For this review, take the finished solid that the model builds, in its own axes (mm). A direction names the side the tool comes from. Coordinates: 2 decimals unless noted, no trailing zeros. Loops run counter-clockwise (first coordinate to the right, second up) from the corner with the lowest first, then second, coordinate; pieces in that order, holes last. Notation, with made-up numbers: (89.5, 70) - (125.5, 70) arc R17 cw to (125.5, 74) - close; hole circle Ø7 at (77.5, -6.75). An arc over 180 degrees is marked (long way). Answer as a JSON object with one key per item and string values. Group by question number.
Item 1: We need section A-A (z = -15). Give the boundary of the cut face in (x, y), then the cut area to 3 significant figures.
Item 2: We need section B-B (y = -7.75). Give the boundary of the cut face in (x, z), then the cut area to 3 significant figures.
Item 3: We need section C-C (z = -23). Give the boundary of the cut face in (x, y), then the cut area to 3 significant figures.
Item 4: Clearance check with a flat-ended pin moving along its axis: pin 1 (5 mm diameter, centred on x = 4, y = 3, fed in from -Z). State where the tip first meets the part, or that it passes through.
Item 5: Tool access review of faces 4 (the flat face through (-3.77, -0.18, -6.44)), 5 (the flat face through (-2.15, -0.18, -18.96)), 6 (the flat face through (-9, 0, -25.4)): name each direction out of +Z, -Z, +X, -X, +Y, -Y from which nothing blocks a thin tool from reaching the whole face with its end or side.
Item 6: To check wall thickness, follow line 1 (X direction, y = -1, z = -9.25); line 2 (X direction, y = -8.25, z = -7.75). State the ranges of each line that lie inside material, in increasing order.
Item 7: Mouldability with a two-part tool opening along X and no side actions: class faces 1 (the flat face through (-0.2, -12.7, -12.5)), 2 (the flat face through (-6.3, -0.2, -6.3)), 3 (the flat face through (12.7, 0, -13)) as released by +X, released by -X, zero draft, split by the parting line, or undercut.
Item 8: We need section D-D (x = 2.25). Give the boundary of the cut face in (y, z).
from build123d import *

# Parameters (mm, degrees)
F0_W     = 25.4
F0_H     = 25.4
F1_DEPTH = 25.4
F3_DEPTH = 25.4
F5_DEPTH = 25.4


with BuildPart() as f1:
    # F0 (on Top) → F1 (new body)
    with BuildSketch(Plane.XY):
        Rectangle(F0_W, F0_H)
    extrude(amount=-F1_DEPTH)

    # F2 (on face) → F3 (cut)
    with BuildSketch(Plane.XZ.offset(12.7)):
        Polygon((0, -12.7), (-4.361447, -25.4), (4.060659, -25.4), align=None)
    extrude(amount=-F3_DEPTH, mode=Mode.SUBTRACT)

    # F4 (on face) → F5 (cut)
    with BuildSketch(Plane.XZ.offset(12.7)):
        Polygon((-2.54, 0), (-7.62, 0), (-4.963026, -12.7), align=None)
    extrude(amount=-F5_DEPTH, mode=Mode.SUBTRACT)


solid = f1.part
Check sheet entries:
{
 "1": {"outline": "(-12.7, -12.7) - (-0.79, -12.7) - (-0.79, 12.7) - (-12.7, 12.7) - close; (0.74, -12.7) - (12.7, -12.7) - (12.7, 12.7) - (0.74, 12.7) - close", "area": "606 mm2"},
 "2": {"outline": "(-12.7, -25.4) - (-4.36, -25.4) - (0, -12.7) - (4.06, -25.4) - (12.7, -25.4) - (12.7, 0) - (-2.54, 0) - (-4.96, -12.7) - (-7.62, 0) - (-12.7, 0) - close", "area": "559 mm2"},
 "3": {"outline": "(-12.7, -12.7) - (-3.54, -12.7) - (-3.54, 12.7) - (-12.7, 12.7) - close; (3.29, -12.7) - (12.7, -12.7) - (12.7, 12.7) - (3.29, 12.7) - close", "area": "472 mm2"},
 "4": {"pin 1": "stops at z = -25.4"},
 "5": {"face 4": "+Z, +Y, -Y", "face 5": "-Z, +Y, -Y", "face 6": "-Z, +X, -X, +Y, -Y"},
 "6": {"line 1": "x = -12.7 to -5.68, -4.3 to 12.7", "line 2": "x = -12.7 to -6, -4.02 to 12.7"},
 "7": {"face 1": "zero draft", "face 2": "undercut", "face 3": "released by +X"},
 "8": {"outline": "(-12.7, -19.74) - (12.7, -19.74) - (12.7, 0) - (-12.7, 0) - close"}
}
